Design review of the part built by this model. Coordinates are the model's own, in mm. Coordinates: 2 decimals unless noted, no trailing zeros. Loops run counter-clockwise (first coordinate to the right, second up) from the corner with the lowest first, then second, coordinate; pieces in that order, holes last. Notation, with made-up numbers: (48, 27) -> (68, 27) arc R17 cw to (68, 51) -> close; hole circle Ø11 at (-35.75, 85). An arc over 180 degrees is marked (long way). One line per item, written item: value. Start each with the question number.
1. For probe 1 along X at (y, z) = (1.55, 0.5); probe 2 along X at (y, z) = (2.5, -21.59); probe 3 along Z at (x, y) = (-58, 2.6), list the stretches that pass through material, from the lowest coordinate up.
2. Add section D-D on z = 57. Write out the cut boundary in (x, y) (3 decimals).
3. Draft analysis for pull direction Z (two halves, no side actions). For faces 1 (the cylindrical face through (-26, 2, -52)), 2 (the flat face through (-73.917, 2, 0)), state which applies: pulls with the +Z half, pulls with the -Z half, needs draft (parallel to the pull), parting line crosses it, or undercut.
4. Insertion check: pin 1 (2 mm diameter, centred on x = -34.29, z = 21.59, fed in from -Y); pin 2 (4.5 mm diameter, centred on x = -38.1, z = -42.418, fed in from +Y) (3 decimals); pin 3 (1 mm diameter, centred on y = 2, z = -27.5, fed in from -X); pin 4 (1 mm diameter, centred on x = -42.5, y = 2.5, fed in from -Z). Each pin has a flat end and moves straight along its axis. Give the tip position at first contact, or say it passes through.
5. Add section A-A on z = 1. Write out the cut boundary in (x, y) (3 decimals), plus the area to 3 significant figures.
6. Add section B-B on x = 8. Write out the cut boundary in (y, z) (3 decimals), plus the area to 3 significant figures.
7. Add section C-C on y = 1.9. Give the number of separate pieces and of enclosed holes in the cut face, plus the area to 3 significant figures.
```python
from build123d import *

# Parameters (mm, degrees)
SKETCH1_R           = 1.651
SKETCH1_W           = 50.8
SKETCH1_H           = 6.35
SKETCH1_W_2         = 6.35
SKETCH1_H_2         = 25.4
BOSS_EXTRUDE1_DEPTH = 3.175


with BuildPart() as part:
    # Sketch1 → Boss-Extrude1 (new body)
    with BuildSketch(Plane(origin=(0, 0, 0), x_dir=(1, 0, 0), z_dir=(0, 1, 0))):
        with BuildLine():
            Line((-73.916912814, 12.7), (-73.916912814, -12.7))
            ThreePointArc((-73.916912814, -12.7), (75, 0), (-73.916912814, 12.7))
        make_face()
        with Locations(Location((-34.29, 21.59, 0), (0, 0, 270))):
            Circle(SKETCH1_R, mode=Mode.SUBTRACT)
        with Locations(Location((34.29, 21.59, 0), (0, 0, 270))):
            Circle(SKETCH1_R, mode=Mode.SUBTRACT)
        with Locations(Location((-34.29, -21.59, 0), (0, 0, 270))):
            Circle(SKETCH1_R, mode=Mode.SUBTRACT)
        with Locations(Location((34.29, -21.59, 0), (0, 0, 270))):
            Circle(SKETCH1_R, mode=Mode.SUBTRACT)
        with Locations(Location((38.1, -42.418, 0), (0, 0, 270))):
            Circle(SKETCH1_R, mode=Mode.SUBTRACT)
        with Locations(Location((-38.1, -42.418, 0), (0, 0, 270))):
            Circle(SKETCH1_R, mode=Mode.SUBTRACT)
        with Locations(Location((-58.676912814, -34.29, 0), (0, 0, 270))):
            Circle(SKETCH1_R, mode=Mode.SUBTRACT)
        with Locations(Location((-58.676912814, 34.29, 0), (0, 0, 270))):
            Circle(SKETCH1_R, mode=Mode.SUBTRACT)
        with Locations(Location((-38.1, 42.418, 0), (0, 0, 270))):
            Circle(SKETCH1_R, mode=Mode.SUBTRACT)
        with Locations(Location((38.1, 42.418, 0), (0, 0, 270))):
            Circle(SKETCH1_R, mode=Mode.SUBTRACT)
        with Locations(Location((12.7, -67.593386492, 0), (0, 0, 90))):
            Circle(SKETCH1_R, mode=Mode.SUBTRACT)
        with Locations(Location((12.7, -34.743386492, 0), (0, 0, 90))):
            Circle(SKETCH1_R, mode=Mode.SUBTRACT)
        with Locations(Location((12.7, 34.743386492, 0), (0, 0, 270))):
            Circle(SKETCH1_R, mode=Mode.SUBTRACT)
        with Locations(Location((12.7, 67.593386492, 0), (0, 0, 270))):
            Circle(SKETCH1_R, mode=Mode.SUBTRACT)
        with Locations(Location((-27.425, -51.168386492, 0), (0, 0, 270))):
            Circle(SKETCH1_R, mode=Mode.SUBTRACT)
        with Locations(Location((-12.7, -34.743386492, 0), (0, 0, 270))):
            Circle(SKETCH1_R, mode=Mode.SUBTRACT)
        with Locations(Location((-12.7, -67.593386492, 0), (0, 0, 270))):
            Circle(SKETCH1_R, mode=Mode.SUBTRACT)
        with Locations(Location((-12.7, 67.593386492, 0), (0, 0, 90))):
            Circle(SKETCH1_R, mode=Mode.SUBTRACT)
        with Locations(Location((-27.425, 51.168386492, 0), (0, 0, 90))):
            Circle(SKETCH1_R, mode=Mode.SUBTRACT)
        with Locations(Location((-12.7, 34.743386492, 0), (0, 0, 90))):
            Circle(SKETCH1_R, mode=Mode.SUBTRACT)
        with Locations((0, 28.575)):
            Rectangle(SKETCH1_W, SKETCH1_H, mode=Mode.SUBTRACT)
        with Locations((41.275, 0)):
            Rectangle(SKETCH1_W_2, SKETCH1_H_2, mode=Mode.SUBTRACT)
        with Locations((0, -28.575)):
            Rectangle(SKETCH1_W, SKETCH1_H, mode=Mode.SUBTRACT)
        with Locations((-41.275, 0)):
            Rectangle(SKETCH1_W_2, SKETCH1_H_2, mode=Mode.SUBTRACT)
    extrude(amount=BOSS_EXTRUDE1_DEPTH)


solid = part.part
```
Worked answers:
1. probe 1: x = -73.92 to -44.45, -38.1 to 38.1, 44.45 to 75
1. probe 2: x = -71.83 to -35.94, -32.64 to 32.64, 35.94 to 71.83
1. probe 3: z = -47.55 to -35.8, -32.78 to 32.78, 35.8 to 47.55
2. outline: (-48.744, 0) -> (48.744, 0) -> (48.744, 3.175) -> (-48.744, 3.175) -> close
3. face 1: undercut
3. face 2: needs draft
4. pin 1: passes through
4. pin 2: stops at y = 3.175
4. pin 3: stops at x = -69.97
4. pin 4: stops at z = -62.14
5. outline: (-73.917, 0) -> (-44.45, 0) -> (-44.45, 3.175) -> (-73.917, 3.175) -> close; (-38.1, 0) -> (38.1, 0) -> (38.1, 3.175) -> (-38.1, 3.175) -> close; (44.45, 0) -> (74.993, 0) -> (74.993, 3.175) -> (44.45, 3.175) -> close
5. area: 432 mm²
6. outline: (0, -74.572) -> (3.175, -74.572) -> (3.175, -31.75) -> (0, -31.75) -> close; (0, -25.4) -> (3.175, -25.4) -> (3.175, 25.4) -> (0, 25.4) -> close; (0, 31.75) -> (3.175, 31.75) -> (3.175, 74.572) -> (0, 74.572) -> close
6. area: 433 mm²
7. separate pieces: 1
7. enclosed holes: 24
7. area: 16,500 mm²
